Verification items for the finished model (mm, model axes). A direction names the side the tool comes from. Coordinates: 2 decimals unless noted, no trailing zeros. Order: outer loops, then holes, each group sorted by start corner. A loop starts at its lowest first (then second) coordinate and runs counter-clockwise, first axis right, second up. Notation, with made-up numbers: (55.25, 39.5) -> (102.25, 39.5) arc R24 ccw to (102.25, 74.5) -> close; hole circle Ø6 at (61, 28.5). An arc over 180 degrees is marked (long way). Use CSV: the item, a comma, the result in double quotes. Start each with the question number.
1) Sectioned sample at A-A on x = -11. Record the boundary of the cut face in (y, z), then the cut area to 3 significant figures.
2) Scan lines: line 1 along Z through (x, y) = (-10.5, -0.75); line 2 along Z through (x, y) = (-30, -3); line 3 along X through (y, z) = (-5.25, -38.5). Record each from-to range of solid material in increasing order.
3) Sectioned sample at B-B on z = -44. Record the boundary of the cut face in (x, y).
4) Tool access check on faces 4 (the cylindrical face through (-40.05, -3.22, -51.82)), 5 (the cylindrical face through (-28.151, -3.212, 1.352)). Record the directions out of +Z, -Z, +X, -X, +Y, -Y that give a thin tool (end or side, any length) a straight path to the whole face; none if there is none.
5) Release check for a two-part mould opening along Z. For faces 1 (the flat face through (-40.627, -3, -29)), 2 (the conical face through (0.455, -0.201, 1.056)), 3 (the flat face through (11.861, -0.258, -54.624)) record: released by +Z, released by -Z, zero draft, split by the parting line, or undercut.
from build123d import *

# Parameters (mm, degrees)
SKETCH1_W     = 1.5875
SKETCH1_H     = 6.35
FILLET1_R     = 3.175
CHAMFER1_SIZE = 0.508


with BuildPart() as part:
    # Sweep1: sweep along a path in Sketch2
    with BuildLine(Plane(origin=(0, 0, 0), x_dir=(1, 0, 0), z_dir=(0, 1, 0))) as sweep1_path:
        Line((0, 0), (-27.6098, 0))
        Line((-27.6098, 0), (-34.045051536, 6.435251536))
        Line((-34.045051536, 6.435251536), (-40.6273, 25.4))
        Line((-40.6273, 25.4), (-40.6273, 31.75))
        Line((-40.6273, 31.75), (-40.270978863, 51.933561137))
        Line((-40.270978863, 51.933561137), (-36.8046, 55.39994))
        Line((-36.8046, 55.39994), (9.1948, 55.39994))
        Line((9.1948, 55.39994), (12.661178863, 51.933561137))
        Line((12.661178863, 51.933561137), (13.0175, 31.75))
        Line((13.0175, 31.75), (13.0175, 25.4))
        Line((13.0175, 25.4), (6.435251536, 6.435251536))
        Line((6.435251536, 6.435251536), (0, 0))
    # Sketch1 → Sweep1 (sweep)
    with BuildSketch(Plane(origin=(0, 0, 0), x_dir=(0, 0, -1), z_dir=(1, 0, 0))):
        with Locations((-0.79375, -3.175)):
            Rectangle(SKETCH1_W, SKETCH1_H)
    sweep(path=sweep1_path.line, transition=Transition.RIGHT)

    # Fillet1
    fillet1_edges = [part.edges().sort_by_distance(p)[0] for p in [
        (7.815488456, -3.175, -5.570424426),
        (6.435251536, -3.175, -6.435251536),
        (-42.2148, -3.175, -25.132338463),
        (-40.6273, -3.175, -25.4),
        (-27.6098, -3.175, 0),
        (14.605, -3.175, -25.132338463),
        (13.0175, -3.175, -25.4),
        (-42.2148, -3.175, -31.764011792),
        (-28.26736403, -3.175, 1.5875),
        (-40.6273, -3.175, -31.75),
        (0.65756403, -3.175, 1.5875),
        (0, -3.175, 0),
        (14.605, -3.175, -31.764011792),
        (13.0175, -3.175, -31.75),
        (-41.846913397, -3.175, -52.602690633),
        (-40.270978863, -3.175, -51.933561137),
        (14.237113397, -3.175, -52.602690633),
        (12.661178863, -3.175, -51.933561137),
        (-37.46216403, -3.175, -56.98744),
        (-36.8046, -3.175, -55.39994),
        (9.85236403, -3.175, -56.98744),
        (9.1948, -3.175, -55.39994),
        (-35.425288456, -3.175, -5.570424426),
        (-34.045051536, -3.175, -6.435251536),
    ]]
    fillet(fillet1_edges, radius=FILLET1_R)

    # Chamfer1
    chamfer1_edges = [part.edges().sort_by_distance(p)[0] for p in [
        (-39.666104179, -6.35, -54.783499851),
        (-39.666104179, 0, -54.783499851),
        (-37.362055867, 0, -56.745757516),
        (-41.617523848, 0, -52.505293622),
        (-42.042174838, 0, -41.542243119),
        (-42.042174838, 0, -41.542243119),
        (-41.617523848, 0, -52.505293622),
        (-42.042174838, -6.35, -41.542243119),
        (-42.042174838, -6.35, -41.542243119),
        (-41.617523848, -6.35, -52.505293622),
        (-37.362055867, -6.35, -56.745757516),
        (-41.617523848, -6.35, -52.505293622),
        (-42.2148, 0, -28.715836665),
        (-42.170610697, 0, -25.139789031),
        (-42.2148, 0, -28.715836665),
        (-42.2148, -6.35, -28.715836665),
        (-42.170610697, -6.35, -25.139789031),
        (-42.2148, -6.35, -28.715836665),
        (-38.851780138, 0, -15.442818824),
        (-35.355298477, 0, -5.614278659),
        (-42.170610697, 0, -25.139789031),
        (-38.851780138, -6.35, -15.442818824),
        (-35.355298477, -6.35, -5.614278659),
        (-42.170610697, -6.35, -25.139789031),
        (-32.053589323, 0, -2.198725293),
        (-28.167255867, 0, 1.345817516),
        (-35.355298477, 0, -5.614278659),
        (-32.053589323, -6.35, -2.198725293),
        (-28.167255867, -6.35, 1.345817516),
        (-35.355298477, -6.35, -5.614278659),
        (-13.8049, -6.35, -56.98744),
        (-13.8049, 0, -56.98744),
        (9.752255867, 0, -56.745757516),
        (-37.362055867, 0, -56.745757516),
        (9.752255867, -6.35, -56.745757516),
        (-37.362055867, -6.35, -56.745757516),
        (12.056304179, -6.35, -54.783499851),
        (12.056304179, 0, -54.783499851),
        (14.007723848, 0, -52.505293622),
        (9.752255867, 0, -56.745757516),
        (14.007723848, -6.35, -52.505293622),
        (9.752255867, -6.35, -56.745757516),
        (14.605, -6.35, -28.715836665),
        (14.605, 0, -28.715836665),
        (14.560810697, 0, -25.139789031),
        (14.605, 0, -28.715836665),
        (14.432374838, 0, -41.542243119),
        (14.007723848, 0, -52.505293622),
        (14.432374838, 0, -41.542243119),
        (14.432374838, -6.35, -41.542243119),
        (14.007723848, -6.35, -52.505293622),
        (14.432374838, -6.35, -41.542243119),
        (14.560810697, -6.35, -25.139789031),
        (14.605, -6.35, -28.715836665),
        (11.241980138, -6.35, -15.442818824),
        (11.241980138, 0, -15.442818824),
        (7.745498477, 0, -5.614278659),
        (14.560810697, 0, -25.139789031),
        (7.745498477, -6.35, -5.614278659),
        (14.560810697, -6.35, -25.139789031),
        (4.443789323, -6.35, -2.198725293),
        (4.443789323, 0, -2.198725293),
        (0.557455867, 0, 1.345817516),
        (7.745498477, 0, -5.614278659),
        (0.557455867, -6.35, 1.345817516),
        (7.745498477, -6.35, -5.614278659),
        (-13.8049, 0, 1.5875),
        (-13.8049, -6.35, 1.5875),
        (-28.167255867, 0, 1.345817516),
        (0.557455867, 0, 1.345817516),
        (-28.167255867, -6.35, 1.345817516),
        (0.557455867, -6.35, 1.345817516),
    ]]
    chamfer(chamfer1_edges, length=CHAMFER1_SIZE)


solid = part.part
Answers follow:
1,outline,"(-6.35, -56.48) -> (-5.84, -56.99) -> (-0.51, -56.99) -> (0, -56.48) -> (0, -55.4) -> (-6.35, -55.4) -> close; (-6.35, 0) -> (0, 0) -> (0, 1.08) -> (-0.51, 1.59) -> (-5.84, 1.59) -> (-6.35, 1.08) -> close"
1,area,"19.6 mm²"
2,line 1,"z = -56.99 to -55.4, 0 to 1.59"
2,line 2,"z = -56.99 to -55.4, -2.39 to -0.15"
2,line 3,"x = -42.1 to -40.51, 12.9 to 14.49"
3,outline,"(-42, -5.84) -> (-41.49, -6.35) -> (-40.41, -6.35) -> (-40.41, 0) -> (-41.49, 0) -> (-42, -0.51) -> close; (12.8, -6.35) -> (13.88, -6.35) -> (14.39, -5.84) -> (14.39, -0.51) -> (13.88, 0) -> (12.8, 0) -> close"
4,face 4,"+Y, -Y"
4,face 5,"+Z, -X, +Y, -Y"
5,face 1,"undercut"
5,face 2,"released by +Z"
5,face 3,"released by -Z"
